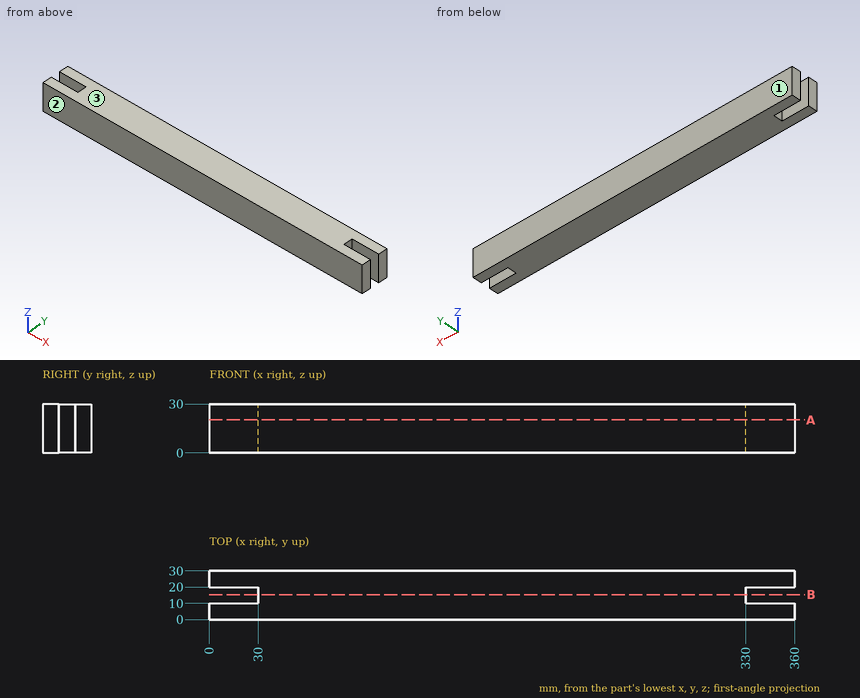
Print and shaded views of the part. All mm, measured from the part's lowest x, y and z. Coordinates: 2 decimals unless noted, no trailing zeros. Loops run counter-clockwise (first coordinate to the right, second up) from the corner with the lowest first, then second, coordinate; pieces in that order, holes last. Notation, with made-up numbers: M 15,-33 L 49,-33 A8 cw 49,-29 Z; hole C -33,58.5 d7. An arc over 180 degrees is marked long. Use a Markdown table: item, result. Add a question column.
Q1. Probe L1, parallel to Y at x = 344.5, z = 20.75; L2, parallel to X at y = 10.5, z = 21.5. List the from-to ranges inside material, lowest first.
Q2. Cut at B-B (y = 15.25). Write the cut outline in (x, z), and give its area (3 significant figures).
Q3. Cut at A-A (z = 20.25). Write the cut outline in (x, y), and give its area (3 significant figures).
Q4. Mould opens along Y. For the marked faces 1, 2 and 3 say: +Y half, -Y half, draft (parallel to the pull), parting line (faces both ways), or undercut.
Worked out:
| question | item | result |
|---|---|---|
| 1 | L1 | y = 0 to 10, 20 to 30 |
| 1 | L2 | x = 30 to 330 |
| 2 | outline | M 30,0 L 330,0 L 330,30 L 30,30 Z |
| 2 | area | 9,000 mm2 |
| 3 | outline | M 0,0 L 360,0 L 360,10 L 330,10 L 330,20 L 360,20 L 360,30 L 0,30 L 0,20 L 30,20 L 30,10 L 0,10 Z |
| 3 | area | 10,200 mm2 |
| 4 | face 1 | +Y half |
| 4 | face 2 | -Y half |
| 4 | face 3 | draft |
